The figure shows three views and two pictorial views of one solid part (mm, origin at its lowest corner). Answer the questions. Coordinates: 2 decimals unless noted, no trailing zeros. Loops run counter-clockwise (first coordinate to the right, second up) from the corner with the lowest first, then second, coordinate; pieces in that order, holes last. Notation, with made-up numbers: M -13,71 L -4,71 A8 cw -4,86 Z; hole C 31,-33 d11. An arc over 180 degrees is marked long. Write each question's results on one line, items separated by ' | '.
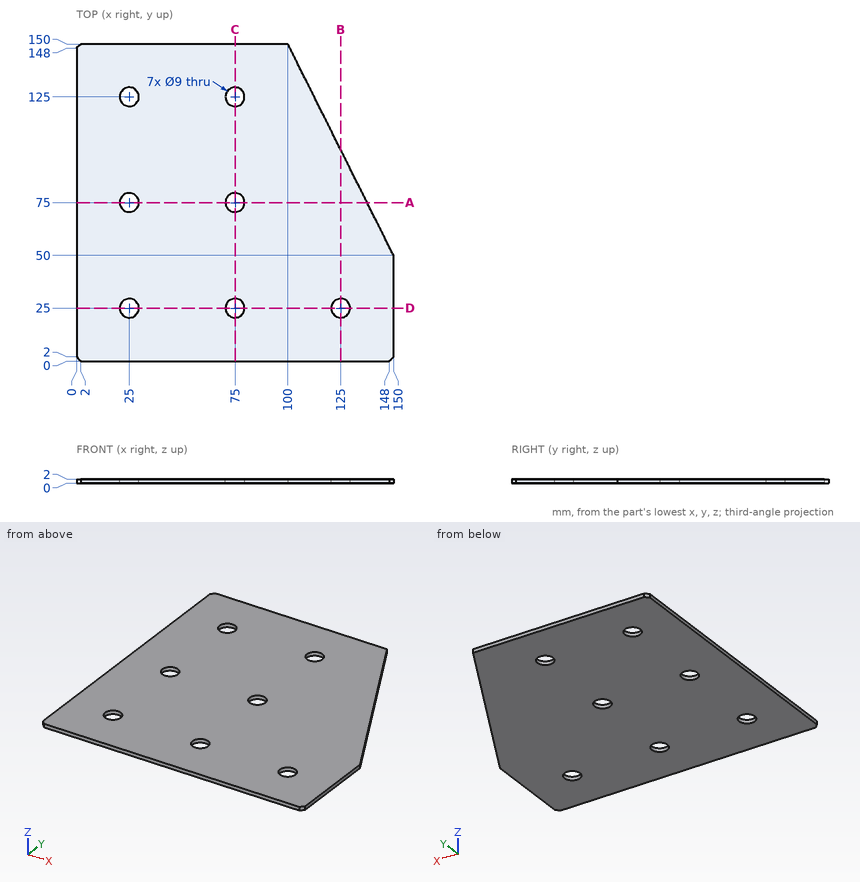
1) Find section A-A, the plane y = 75. Give the vertices of the cut face in (x, z).
Check result:
outline: M 0,0 L 20.5,0 L 20.5,2 L 0,2 Z; M 29.5,0 L 70.5,0 L 70.5,2 L 29.5,2 Z; M 79.5,0 L 137.5,0 L 137.5,2 L 79.5,2 Z
2) Find section B-B, the plane x = 125. Give the vertices of the cut face in (y, z).
Check result:
outline: M 0,0 L 20.5,0 L 20.5,2 L 0,2 Z; M 29.5,0 L 100,0 L 100,2 L 29.5,2 Z
3) Find section C-C, the plane x = 75. Give the vertices of the cut face in (y, z).
Check result:
outline: M 0,0 L 20.5,0 L 20.5,2 L 0,2 Z; M 29.5,0 L 70.5,0 L 70.5,2 L 29.5,2 Z; M 79.5,0 L 120.5,0 L 120.5,2 L 79.5,2 Z; M 129.5,0 L 150,0 L 150,2 L 129.5,2 Z
4) Straight lines are drawn through the part: probe 1 along Y at (x, z) = (25, 1.2); probe 2 along X at (y, z) = (74.5, 1.6). For each, find the intervals that lie inside material, in ascending order. Write a range as [from, to].
Check result:
probe 1: [0, 20.5], [29.5, 70.5], [79.5, 120.5], [129.5, 150] | probe 2: [0, 20.53], [29.47, 70.53], [79.47, 137.75]
